```python
from build123d import *

# Parameters (mm, degrees)
BOSS_EXTRUDE1_DEPTH        = 20
CHAMFER1_SIZE              = 10
CHAMFER2_SIZE              = 10
CHAMFER2_SIZE2             = 22.460367739
FILLET2_R                  = 10
FILLET3_R                  = 5
F_8_5_8_5_DIAMETER_HOLE1_D = 8.5
SKETCH6_R                  = 7
CUT_EXTRUDE1_DEPTH         = 10
SKETCH7_R                  = 22.103989718
SKETCH7_R_2                = 10.5
CUT_EXTRUDE2_DEPTH         = 9


with BuildPart() as part:
    # Sketch1 → Boss-Extrude1 (new body)
    with BuildSketch(Plane(origin=(0, 0, 0), x_dir=(0, 0, -1), z_dir=(1, 0, 0))):
        with BuildLine():
            Line((-35.628848893, 0), (35.628848893, 0))
            Line((35.628848893, 0), (35.628848893, -30))
            Line((35.628848893, -30), (23.628848893, -30))
            ThreePointArc((23.628848893, -30), (4.632142534, -7.808067016), (-21.431810469, -21))
            Line((-21.431810469, -21), (-24.628848893, -21))
            Line((-24.628848893, -21), (-24.628848893, -30))
            Line((-24.628848893, -30), (-48.083267238, -30))
            Line((-48.083267238, -30), (-48.083267238, 0))
            Line((-48.083267238, 0), (-35.628848893, 0))
        make_face()
    extrude(amount=BOSS_EXTRUDE1_DEPTH)

    # Chamfer1
    chamfer1_edges = [part.edges().sort_by_distance(p)[0] for p in [
        (10, 0, -35.628848893),
    ]]
    chamfer(chamfer1_edges, length=CHAMFER1_SIZE)

    # Chamfer2
    chamfer2_edges = [part.edges().sort_by_distance(p)[0] for p in [
        (10, 0, 48.083267238),
    ]]
    chamfer2_side = [part.faces().sort_by_distance(p)[0] for p in [
        (10, -15, 48.083267238),
    ]]
    chamfer(chamfer2_edges, length=CHAMFER2_SIZE, length2=CHAMFER2_SIZE2, reference=chamfer2_side[0])

    # Fillet2
    fillet2_edges = [part.edges().sort_by_distance(p)[0] for p in [
        (10, 0, -25.628848893),
        (10, 0, 25.622899499),
    ]]
    fillet(fillet2_edges, radius=FILLET2_R)

    # Fillet3
    fillet3_edges = [part.edges().sort_by_distance(p)[0] for p in [
        (10, -21, 21.431810469),
    ]]
    fillet(fillet3_edges, radius=FILLET3_R)

    # Ø8.5 (8.5) Diameter Hole1 (through all)
    with Locations(Plane(origin=(0, -30, 0), x_dir=(-1, 0, 0), z_dir=(0, -1, 0))):
        with Locations((-10, -35.856058066), (-10, 29.628848893)):
            Hole(F_8_5_8_5_DIAMETER_HOLE1_D / 2)

    # Sketch6 → Cut-Extrude1 (cut)
    with BuildSketch(Plane(origin=(0, 0, 0), x_dir=(1, 0, 0), z_dir=(0, 1, 0))):
        with Locations(Location((10, -35.856058066, 0), (0, 0, 270))):
            Circle(SKETCH6_R)
        with Locations((10, 29.628848893)):
            Circle(SKETCH6_R)
    extrude(amount=-CUT_EXTRUDE1_DEPTH, mode=Mode.SUBTRACT)

    # Sketch7 → Cut-Extrude2 (cut)
    with BuildSketch(Plane.XZ.offset(30)):
        with Locations((10, 35.856058066)):
            Circle(SKETCH7_R)
        with Locations((10, 35.856058066)):
            Circle(SKETCH7_R_2, mode=Mode.SUBTRACT)
    extrude(amount=-CUT_EXTRUDE2_DEPTH, mode=Mode.SUBTRACT)


solid = part.part
```
The listing builds one solid part. Answer for the finished solid, in the listing's coordinates (mm). A direction names the side the tool comes from. Give positions to 0.01 mm unless a question says otherwise; leave off trailing zeros. Order: outer loops, then holes, each group sorted by start corner. A loop starts at its lowest first (then second) coordinate and runs counter-clockwise, first axis right, second up. Notation, with made-up numbers: M 81,-23 L 97,-23 A8 cw 97,-16 Z; hole C 24,-38.5 d7. An arc over 180 degrees is marked long. Put each result on its own line as item: value. Start each with the question number.
Item 1: The part is cut by section C-C, the plane z = 34. Determine the outline of the cut face in (x, y), and give its area (3 significant figures).
Item 2: For a pull along Z with two mould halves and no side action, classify faces 1 (the face through (9.9, -30, 40.4)), 2 (the face through (9.745, -6.067, -22.633)), 3 (the face through (10.14, -0.007, -21.868)) as +Z half, -Z half, draft (parallel to the pull), parting line (faces both ways), or undercut.
Item 3: The part is cut by section A-A, the plane y = -25. Determine the outline of the cut face in (x, z).
Item 4: Find the intervals of material crossed by line 1 along Z through (x, y) = (10, -14.75); line 2 along Z through (x, y) = (10.5, -22); line 3 along Z through (x, y) = (10, -3.5), in increasing order.
Item 5: The part is cut by section B-B, the plane x = 10. Determine the outline of the cut face in (y, z).
Item 6: Flat-ended cylindrical pins translate along their axes: P1, Ø7, axis at x = 10.5, z = 34.5, coming from the +Y side; P2, Ø1, axis at x = 10.5, y = -8, coming from the -Z side; P3, Ø2, axis at x = 9.5, z = -11.5, coming from the -Y side. Find the tip coordinate at first contact, or state that the pin passes through.
Item 7: The part is cut by section D-D, the plane x = 1.5. Determine the outline of the cut face in (y, z), and give its area (3 significant figures).
Item 8: Which of the six approach directions +Z, -Z, +X, -X, +Y, -Y give full straight-line access (tool end or side, diameter ignored) to faces 4 (the face through (10.185, -25.563, 46.354)), 5 (the face through (10.14, -20.346, 21.938)), 6 (the face through (13, -10, -26))?
Answer key:
1. outline: M 0,-30 L 6.18,-30 L 6.18,-10 L 3.25,-10 L 3.25,-3.73 L 0,-3.73 Z; M 13.82,-30 L 20,-30 L 20,-3.73 L 16.75,-3.73 L 16.75,-10 L 13.82,-10 Z
1. area: 288 mm²
2. face 1: draft
2. face 2: undercut
2. face 3: -Z half
3. outline: M 0,-35.63 L 20,-35.63 L 20,-22.88 L 0,-22.88 Z; M 0,32.65 A10.5 ccw 20,32.65 L 20,39.06 A10.5 ccw 0,39.06 Z; hole C 10,-29.63 d8.5; hole C 10,35.86 d8.5
4. line 1: z = -35.63 to -33.88, -25.38 to -17.18, 17.18 to 31.61, 40.11 to 48.08
4. line 2: z = -35.63 to -33.85, -25.41 to -21.87, 25.37 to 31.64, 40.08 to 46.34
4. line 3: z = -22.63 to 28.86
5. outline: M -30,-35.63 L -10,-35.63 L -10,-33.88 L -30,-33.88 Z; M -30,-25.38 L -10,-25.38 L -10,-22.63 L -0.07,-22.63 A10 ccw 0,-21.49 L 0,23.5 A10 ccw -0.86,27.56 L -1.44,28.86 L -10,28.86 L -10,31.61 L -30,31.61 L -30,25.36 L -21,25.36 L -21,24.41 A5 ccw -18.62,20.15 A23.65 cw -30,-23.63 Z; M -30,40.11 L -10,40.11 L -10,42.86 L -7.67,42.86 L -10,48.08 L -21,48.08 L -21,46.36 L -30,46.36 Z
6. P1: stops at y = -10
6. P2: stops at z = -22.7
6. P3: stops at y = -10.92
7. outline: M -30,-35.63 L -10,-35.63 L -2.93,-28.56 A10 ccw 0,-21.49 L 0,23.5 A10 ccw -0.86,27.56 L -10,48.08 L -21,48.08 L -21,42.02 L -30,42.02 L -30,29.69 L -21,29.69 L -21,24.41 A5 ccw -18.62,20.15 A23.65 cw -30,-23.63 Z
7. area: 1,400 mm²
8. face 4: +Z, -Y
8. face 5: +X, -X, -Y
8. face 6: +Y
